Design review of the part built by this model. Coordinates are the model's own, in mm. A direction names the side the tool comes from. Coordinates: 2 decimals unless noted, no trailing zeros. Loops run counter-clockwise (first coordinate to the right, second up) from the corner with the lowest first, then second, coordinate; pieces in that order, holes last. Notation, with made-up numbers: M 13,-7 L 54,-7 A25 cw 54,29 Z; hole C 85.25,27 d11. An arc over 180 degrees is marked long. Put each result on its own line as item: value. Start each with the question number.
(1) The part is to be moulded in two halves that separate along Z. For faces 3 (the flat face through (-2, 1, 4)), 4 (the flat face through (-24.65, -15.8, 19.28)), 5 (the flat face through (-50, 1, -15)), say which applies: +Z half, -Z half, draft (parallel to the pull), parting line (faces both ways), or undercut.
(2) Clearance check with flat-ended pins moving along their axes: pin 1 (2 mm diameter, centred on x = -44, z = -10, fed in from -Y); pin 2 (4 mm diameter, centred on x = -21.5, z = 10.5, fed in from +Y); pin 3 (19.5 mm diameter, centred on x = -25.5, y = 8.5, fed in from +Z). State where each tip first meets the part, or that it passes through.
(3) Take a section at A-A, the plane x = -24. Give the boundary of the cut face in (y, z).
(4) For faces 1 (the cylindrical face through (-24.65, -5.56, 17.69)), 2 (the flat face through (-26, 2, -14.785)), list the 3-axis set-ups (+Z, -Z, +X, -X, +Y, -Y) from which the entire face can be reached by the end or side of a thin tool; tool diameter is ignored.
(5) Take a section at B-B, the plane y = 7. Give the boundary of the cut face in (x, z), then the cut area to 3 significant figures.
(6) For probe 1 along Z at (x, y) = (-27.5, -6); probe 2 along X at (y, z) = (25, 3.5); probe 3 along Y at (x, z) = (-17, -7), list the stretches that pass through material, from the lowest coordinate up. Write a range as [from, to].
(7) Take a section at C-C, the plane z = 3. Give the boundary of the cut face in (x, y).
```python
from build123d import *

# Parameters (mm, degrees)
F1_DEPTH = 50
F2_DEPTH = 2


with BuildPart() as f1:
    # F0 (on Right) → F1 (new body)
    with BuildSketch(Plane.YZ):
        with BuildLine():
            Line((-18.500151, -15.885202), (21.499849, -15.885202))
            ThreePointArc((21.499849, -15.885202), (28.776178, 4.748888), (18.594223, 24.114798))
            Line((18.594223, 24.114798), (-1.211139, 21.331336))
            ThreePointArc((-1.211139, 21.331336), (-5.644923, 17.678725), (-10.913745, 19.967723))
            Line((-10.913745, 19.967723), (-20.816425, 18.575992))
            ThreePointArc((-20.816425, 18.575992), (-25.786783, 0.933475), (-18.500151, -15.885202))
        make_face()
        with BuildLine():
            ThreePointArc((-18.016041, -14.785202), (-24.689377, 1.008996), (-20.187486, 17.553574))
            Line((-20.187486, 17.553574), (-11.387244, 18.790367))
            ThreePointArc((-11.387244, 18.790367), (-5.491832, 16.589431), (-0.431459, 20.330102))
            Line((-0.431459, 20.330102), (18.271464, 22.958627))
            ThreePointArc((18.271464, 22.958627), (27.678942, 4.670945), (21.015738, -14.785202))
            Line((21.015738, -14.785202), (-18.016041, -14.785202))
        make_face(mode=Mode.SUBTRACT)
    extrude(amount=-F1_DEPTH)

    # F0 (on Right) → F2 (join)
    with BuildSketch(Plane.YZ):
        with BuildLine():
            Line((-11.387244, 18.790367), (-20.187486, 17.553574))
            ThreePointArc((-20.187486, 17.553574), (-24.689377, 1.008996), (-18.016041, -14.785202))
            Line((-18.016041, -14.785202), (21.015738, -14.785202))
            ThreePointArc((21.015738, -14.785202), (27.678942, 4.670945), (18.271464, 22.958627))
            Line((18.271464, 22.958627), (-0.431459, 20.330102))
            ThreePointArc((-0.431459, 20.330102), (-5.491832, 16.589431), (-11.387244, 18.790367))
        make_face()
    extrude(amount=-F2_DEPTH)


solid = f1.part
```
Computed values:
1. face 3: undercut
1. face 4: +Z half
1. face 5: draft
2. pin 1: stops at y = -23.19
2. pin 2: stops at y = 28.24
2. pin 3: stops at z = 24.07
3. outline: M -20.82,18.58 A27.35 ccw -18.5,-15.89 L 21.5,-15.89 A27.35 ccw 18.59,24.11 L -1.21,21.33 A5.5 cw -10.91,19.97 Z; hole M -20.19,17.55 A26.25 ccw -18.02,-14.79 L 21.02,-14.79 A26.25 ccw 18.27,22.96 L -0.43,20.33 A6.6 cw -11.39,18.79 Z
4. face 1: +Z, +X, -X
4. face 2: -X
5. outline: M -50,-15.89 L 0,-15.89 L 0,22.49 L -50,22.49 L -50,21.37 L -2,21.37 L -2,-14.79 L -50,-14.79 Z
5. area: 183 mm^2
6. probe 1: z = [-15.89, -14.79], [16.54, 17.64]
6. probe 2: x = [-2, 0]
6. probe 3: y = [-24.04, -22.86], [25.86, 27.04]
7. outline: M -50,-25.85 L 0,-25.85 L 0,28.85 L -50,28.85 L -50,27.75 L -2,27.75 L -2,-24.75 L -50,-24.75 Z
